Here's how the part is built. I have some questions about the finished solid (model axes, mm). Face numbers are marked on the shaded views. A direction names the side the tool comes from. Give positions to 0.01 mm unless a question says otherwise; leave off trailing zeros. Write each loop counter-clockwise with the first axis right and the second up, starting at its lowest first coordinate (ties: lowest second). Pieces come first, ordered by that corner, then holes. Notation, with made-up numbers: (38.5, 49) -> (48.5, 49) arc R20 cw to (48.5, 71) -> close; hole circle Ø6 at (21.25, 49). An arc over 180 degrees is marked (long way). Use one line per item in the form item = value.
```python
from build123d import *

# Parameters (mm, degrees)
F0_W          = 2.1
F0_H          = 8.055364
F0_H_2        = 10.9
F1_DEPTH      = 2.1
F2_DEPTH      = 50
F2_DEPTH_BACK = 2.1
F3_DEPTH      = 47.9
F4_SIZE       = 5
F5_DEPTH      = 25
F6_SIZE       = 8
F7_R          = 4


with BuildPart() as f1:
    # F0 (on Top) → F1 (new body)
    with BuildSketch(Plane.XY):
        with BuildLine():
            Line((8.642329, -3.944636), (22.9, -3.944636))
            Line((22.9, -3.944636), (22.9, 7.9))
            ThreePointArc((22.9, 7.9), (18.506602, 18.506602), (7.9, 22.9))
            Line((7.9, 22.9), (-7.9, 22.9))
            ThreePointArc((-7.9, 22.9), (-18.506602, 18.506602), (-22.9, 7.9))
            Line((-22.9, 7.9), (-22.9, -3.944636))
            Line((-22.9, -3.944636), (-8.642329, -3.944636))
            ThreePointArc((-8.642329, -3.944636), (-2.0184, 9.283106), (9.5, 0))
            ThreePointArc((9.5, 0), (9.283106, -2.0184), (8.642329, -3.944636))
        make_face()
        with BuildLine():
            Line((-22.9, -22.9), (22.9, -22.9))
            Line((22.9, -22.9), (22.9, -12))
            Line((22.9, -12), (22.9, -3.944636))
            Line((22.9, -3.944636), (8.642329, -3.944636))
            ThreePointArc((8.642329, -3.944636), (0, -9.5), (-8.642329, -3.944636))
            Line((-8.642329, -3.944636), (-22.9, -3.944636))
            Line((-22.9, -3.944636), (-22.9, -12))
            Line((-22.9, -12), (-22.9, -22.9))
        make_face()
        with BuildLine():
            ThreePointArc((-8.642329, -3.944636), (0, -9.5), (8.642329, -3.944636))
            Line((8.642329, -3.944636), (-8.642329, -3.944636))
        make_face()
        with BuildLine():
            Line((22.9, -3.944636), (25, -3.944636))
            Line((25, -3.944636), (25, 10))
            ThreePointArc((25, 10), (20.606602, 20.606602), (10, 25))
            Line((10, 25), (-10, 25))
            ThreePointArc((-10, 25), (-20.606602, 20.606602), (-25, 10))
            Line((-25, 10), (-25, -3.944636))
            Line((-25, -3.944636), (-22.9, -3.944636))
            Line((-22.9, -3.944636), (-22.9, 7.9))
            ThreePointArc((-22.9, 7.9), (-18.506602, 18.506602), (-7.9, 22.9))
            Line((-7.9, 22.9), (7.9, 22.9))
            ThreePointArc((7.9, 22.9), (18.506602, 18.506602), (22.9, 7.9))
            Line((22.9, 7.9), (22.9, -3.944636))
        make_face()
        with BuildLine():
            Line((-8.642329, -3.944636), (8.642329, -3.944636))
            ThreePointArc((8.642329, -3.944636), (9.283106, -2.0184), (9.5, 0))
            ThreePointArc((9.5, 0), (-2.0184, 9.283106), (-8.642329, -3.944636))
        make_face()
        Polygon((-25, -15), (-25, -22.9), (-22.9, -22.9), (-22.9, -12), (-25, -12), (-29.1, -12), (-29.1, -25), (-27, -25), (-27, -15), align=None)
        Polygon((-25, -25), (25, -25), (25, -22.9), (22.9, -22.9), (-22.9, -22.9), (-25, -22.9), align=None)
        with Locations((-23.95, -7.972318)):
            Rectangle(F0_W, F0_H)
        with Locations((23.95, -7.972318)):
            Rectangle(F0_W, F0_H)
        with Locations((23.95, -17.45)):
            Rectangle(F0_W, F0_H_2)
    extrude(amount=-F1_DEPTH)

    # F0 (on Top) → F2 (join, two sides)
    with BuildSketch(Plane.XY) as f2_sk:
        with BuildLine():
            Line((-22.9, -22.9), (22.9, -22.9))
            Line((22.9, -22.9), (22.9, -12))
            Line((22.9, -12), (22.9, -3.944636))
            Line((22.9, -3.944636), (8.642329, -3.944636))
            ThreePointArc((8.642329, -3.944636), (0, -9.5), (-8.642329, -3.944636))
            Line((-8.642329, -3.944636), (-22.9, -3.944636))
            Line((-22.9, -3.944636), (-22.9, -12))
            Line((-22.9, -12), (-22.9, -22.9))
        make_face()
        Polygon((-25, -15), (-25, -22.9), (-22.9, -22.9), (-22.9, -12), (-25, -12), (-29.1, -12), (-29.1, -25), (-27, -25), (-27, -15), align=None)
        Polygon((-25, -25), (25, -25), (25, -22.9), (22.9, -22.9), (-22.9, -22.9), (-25, -22.9), align=None)
        with Locations((23.95, -17.45)):
            Rectangle(F0_W, F0_H_2)
        with Locations((-23.95, -7.972318)):
            Rectangle(F0_W, F0_H)
        with Locations((23.95, -7.972318)):
            Rectangle(F0_W, F0_H)
    extrude(amount=F2_DEPTH)
    extrude(f2_sk.sketch, amount=-F2_DEPTH_BACK)

    # F0 (on Top) → F3 (cut)
    with BuildSketch(Plane.XY):
        with BuildLine():
            Line((-22.9, -22.9), (22.9, -22.9))
            Line((22.9, -22.9), (22.9, -12))
            Line((22.9, -12), (22.9, -3.944636))
            Line((22.9, -3.944636), (8.642329, -3.944636))
            ThreePointArc((8.642329, -3.944636), (0, -9.5), (-8.642329, -3.944636))
            Line((-8.642329, -3.944636), (-22.9, -3.944636))
            Line((-22.9, -3.944636), (-22.9, -12))
            Line((-22.9, -12), (-22.9, -22.9))
        make_face()
        with Locations((-23.95, -7.972318)):
            Rectangle(F0_W, F0_H)
        with Locations((23.95, -7.972318)):
            Rectangle(F0_W, F0_H)
    extrude(amount=F3_DEPTH, mode=Mode.SUBTRACT)

    # F4
    f4_edges = [f1.edges().sort_by_distance(p)[0] for p in [
        (0, -22.9, 47.9),
    ]]
    chamfer(f4_edges, length=F4_SIZE)

    # F0 (on Top) → F5 (join)
    with BuildSketch(Plane.XY):
        with BuildLine():
            Line((22.9, -3.944636), (25, -3.944636))
            Line((25, -3.944636), (25, 10))
            ThreePointArc((25, 10), (20.606602, 20.606602), (10, 25))
            Line((10, 25), (-10, 25))
            ThreePointArc((-10, 25), (-20.606602, 20.606602), (-25, 10))
            Line((-25, 10), (-25, -3.944636))
            Line((-25, -3.944636), (-22.9, -3.944636))
            Line((-22.9, -3.944636), (-22.9, 7.9))
            ThreePointArc((-22.9, 7.9), (-18.506602, 18.506602), (-7.9, 22.9))
            Line((-7.9, 22.9), (7.9, 22.9))
            ThreePointArc((7.9, 22.9), (18.506602, 18.506602), (22.9, 7.9))
            Line((22.9, 7.9), (22.9, -3.944636))
        make_face()
        with Locations((-23.95, -7.972318)):
            Rectangle(F0_W, F0_H)
        with Locations((23.95, -7.972318)):
            Rectangle(F0_W, F0_H)
    extrude(amount=F5_DEPTH)

    # F6
    f6_edges = [f1.edges().sort_by_distance(p)[0] for p in [
        (23.95, -12, 47.9),
        (-23.95, -12, 47.9),
    ]]
    chamfer(f6_edges, length=F6_SIZE)

    # F7
    f7_edges = [f1.edges().sort_by_distance(p)[0] for p in [
        (25, -14.472318, 50),
    ]]
    fillet(f7_edges, radius=F7_R)


solid = f1.part
```
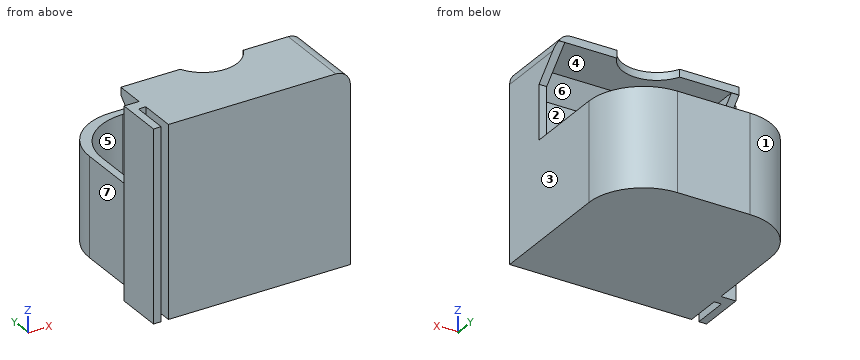
Q1. I want a section at C-C, the plane y = -0.5. Write out the boundary of the cut face in (x, z), and give its area (3 significant figures).
Result set:
outline = (-25, -2.1) -> (25, -2.1) -> (25, 25) -> (22.9, 25) -> (22.9, 0) -> (-22.9, 0) -> (-22.9, 25) -> (-25, 25) -> close
area = 210 mm2
Q2. I want a section at B-B, the plane z = 27. Write out the boundary of the cut face in (x, y).
Result set:
outline = (-29.1, -25) -> (-27, -25) -> (-27, -15) -> (-25, -15) -> (-25, -25) -> (25, -25) -> (25, -12) -> (22.9, -12) -> (22.9, -22.9) -> (-22.9, -22.9) -> (-22.9, -12) -> (-29.1, -12) -> close
Q3. If we mould it in two halves opening along X, with no side actions, what happens to the marked faces 1, 2, 3 and 4? For each: +X half, -X half, draft (parallel to the pull), parting line (faces both ways), or undercut.
Result set:
face_1 = -X half
face_2 = undercut
face_3 = +X half
face_4 = undercut
Q4. Will these pins go through, and if not, where does the flat tip stop? pin 1 Ø12 at (y, z) = (7.5, 12) entering from -X; pin 2 Ø6 at (x, y) = (-19, 7) entering from +Z; pin 3 Ø1 at (x, z) = (-22.5, 33) entering from +Y.
Result set:
pin_1 = -25
pin_2 = 0
pin_3 = -12
Q5. If I drill on line 1 along X through (y, z) = (-18, 44.5); line 2 along X through (y, z) = (-6, 2.5), over which ranges is the centre line in solid material (lowest first)? Write a range as from..to.
Result set:
line_1 = -29.1..-27, -25..-22.9, 22.9..25
line_2 = -25..-22.9, 22.9..25
Q6. I want a section at A-A, the plane z = 18. Write out the boundary of the cut face in (x, y), and give its area (3 significant figures).
Result set:
outline = (-29.1, -25) -> (-27, -25) -> (-27, -15) -> (-25, -15) -> (-25, -25) -> (25, -25) -> (25, 10) arc R15 ccw to (10, 25) -> (-10, 25) arc R15 ccw to (-25, 10) -> (-25, -12) -> (-29.1, -12) -> close; hole (-22.9, -22.9) -> (22.9, -22.9) -> (22.9, 7.9) arc R15 ccw to (7.9, 22.9) -> (-7.9, 22.9) arc R15 ccw to (-22.9, 7.9) -> close
area = 436 mm2
Q7. Which directions (+Z, -Z, +X, -X, +Y, -Y) give clear straight access to the entire face, cutting with the end or side of a thin tool? Please do the marked faces 5, 6 and 7.
Result set:
face_5 = +Z
face_6 = +Y
face_7 = +Z, -Z, -X, +Y
Q8. I want a section at D-D, the plane x = 22. Write out the boundary of the cut face in (y, z), and give its area (3 significant figures).
Result set:
outline = (-25, -2.1) -> (19, -2.1) -> (19, 25) -> (13.02, 25) -> (13.02, 0) -> (-22.9, 0) -> (-22.9, 42.9) -> (-17.9, 47.9) -> (-3.94, 47.9) -> (-3.94, 49.87) -> (-25, 49.87) -> close
area = 397 mm2
